Can you work these out from the model? Positions are in its coordinate system, mm. Coordinates: 2 decimals unless noted, no trailing zeros. Loops run counter-clockwise (first coordinate to the right, second up) from the corner with the lowest first, then second, coordinate; pieces in that order, holes last.
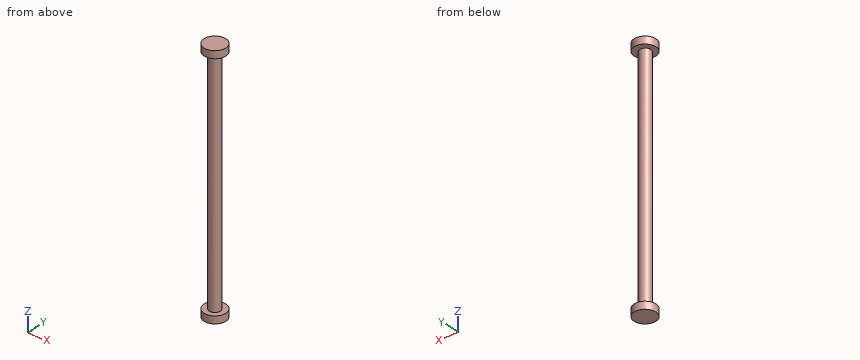
```python
from build123d import *

# Parameters (mm, degrees)
SKETCH_R     = 1.5
PAD_DEPTH    = 32
SKETCH001_R  = 3
PAD001_DEPTH = 2
SKETCH002_R  = 3
PAD002_DEPTH = 2


with BuildPart() as part:
    # Sketch → Pad (new body, symmetric)
    with BuildSketch(Plane.XY):
        with Locations((0.039321, -0.137621)):
            Circle(SKETCH_R)
    extrude(amount=PAD_DEPTH, both=True)

    # Sketch001 (on Face2 of Pad) → Pad001 (join)
    with BuildSketch(Plane(origin=(0, 0, -32), x_dir=(1, 0, 0), z_dir=(0, 0, -1))):
        Circle(SKETCH001_R)
    extrude(amount=PAD001_DEPTH)

    # Sketch002 (on Face5 of Pad001) → Pad002 (join)
    with BuildSketch(Plane.XY.offset(32)):
        Circle(SKETCH002_R)
    extrude(amount=PAD002_DEPTH)


solid = part.part
```
Item 1: Suppose I cut it at C-C, the plane z = 6. Please give me the cut outline in (x, y).
Results are:
outline: circle Ø3 at (0.04, -0.14)
Item 2: Suppose I cut it at B-B, the plane x = -0.2. Please give me the cut outline in (y, z), plus the area to 3 significant figures.
Results are:
outline: (-2.99, -34) - (2.99, -34) - (2.99, -32) - (1.34, -32) - (1.34, 32) - (2.99, 32) - (2.99, 34) - (-2.99, 34) - (-2.99, 32) - (-1.62, 32) - (-1.62, -32) - (-2.99, -32) - close
area: 213 mm2
Item 3: I need wall thicknesses on line 1 along Z through (x, y) = (-0.35, -2.4); line 2 along X through (y, z) = (-1.2, 16.5); line 3 along Y through (x, z) = (-1, -11.5). Which ranges of each line are inside material? Lowest first, please.
Results are:
line 1: z = -34 to -32, 32 to 34
line 2: x = -1.02 to 1.1
line 3: y = -1.22 to 0.94
Item 4: Suppose I cut it at A-A, the plane y = 2.45. Please give me the cut outline in (x, z), plus the area to 3 significant figures.
Results are:
outline: (-1.73, -34) - (1.73, -34) - (1.73, -32) - (-1.73, -32) - close; (-1.73, 32) - (1.73, 32) - (1.73, 34) - (-1.73, 34) - close
area: 13.9 mm2
